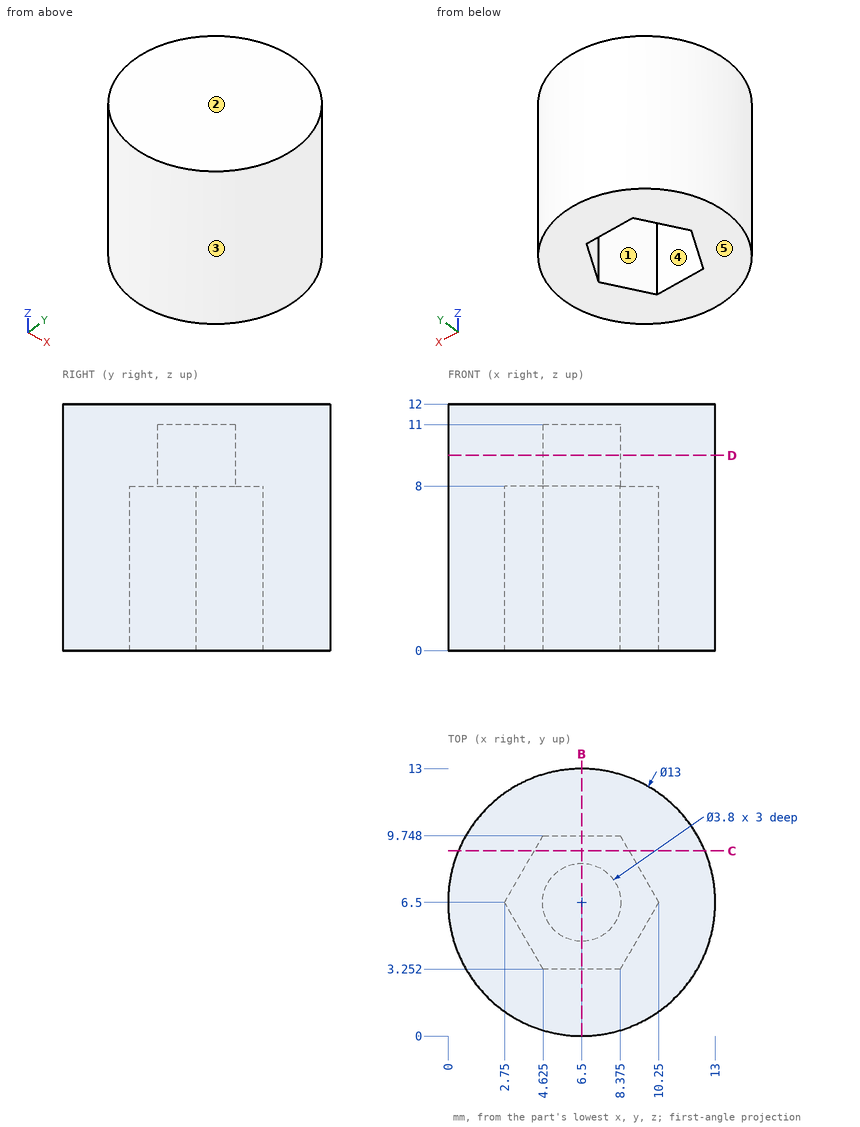
Job drawing, mm, ordinate dimensions from the low corner. One solid piece. A direction names the side the tool comes from. Coordinates: 2 decimals unless noted, no trailing zeros. Order: outer loops, then holes, each group sorted by start corner. A loop starts at its lowest first (then second) coordinate and runs counter-clockwise, first axis right, second up. Notation, with made-up numbers: (81.25, -32.75) - (127.25, -32.75) arc R30 cw to (127.25, -1.75) - close; hole circle Ø10 at (62.5, -12.75). An arc over 180 degrees is marked (long way). Return JSON: item names as keys, results as strings. Group by question number.
1) Flat gauge pins, fed straight in: P1, Ø6, axis at y = 11, z = 8.5, coming from the +X side (1 decimal); P2, Ø4, axis at x = 6.5, y = 6, coming from the -Z side; P3, Ø3, axis at x = 9, z = 4.5, coming from the -Y side. Where does each tip first touch, or does it go through?
2) Mould opens along Y. For the marked faces 1, 2 and 3 say: released by +Y, released by -Y, zero draft, split by the parting line, or undercut.
3) Probe line 1 (Y direction, x = 6.25, z = 3.25) (1 decimal); line 2 (Y direction, x = 6.5, z = 9); line 3 (Z direction, x = 8, y = 7). List the from-to ranges inside material, lowest first. Write a range as from..to.
4) Saw through at D-D, the plane z = 9.5. Write the cut outline in (x, y), plus the area to 3 significant figures.
5) Saw through at B-B, the plane x = 6.5. Write the cut outline in (y, z).
6) Tool access for the marked faces 4 and 5: list every direction of +Z, -Z, +X, -X, +Y, -Y with a clear straight run to the whole face (end or side of a thin tool).
7) Saw through at C-C, the plane y = 9. Write the cut outline in (x, z), plus the area to 3 significant figures.
Values found:
{
 "1": {"P1": "stops at x = 12.8", "P2": "stops at z = 8", "P3": "stops at y = 0.08"},
 "2": {"face 1": "undercut", "face 2": "zero draft", "face 3": "split by the parting line"},
 "3": {"line 1": "y = 0..3.3, 9.7..13", "line 2": "y = 0..4.6, 8.4..13", "line 3": "z = 11..12"},
 "4": {"outline": "circle Ø13 at (6.5, 6.5); hole circle Ø3.8 at (6.5, 6.5)", "area": "121 mm²"},
 "5": {"outline": "(0, 0) - (3.25, 0) - (3.25, 8) - (4.6, 8) - (4.6, 11) - (8.4, 11) - (8.4, 8) - (9.75, 8) - (9.75, 0) - (13, 0) - (13, 12) - (0, 12) - close"},
 "6": {"face 4": "-Z", "face 5": "-Z, +X, -X, +Y, -Y"},
 "7": {"outline": "(0.5, 0) - (4.19, 0) - (4.19, 8) - (8.81, 8) - (8.81, 0) - (12.5, 0) - (12.5, 12) - (0.5, 12) - close", "area": "107 mm²"}
}
